Source: CAD feature listing. Evaluate the final solid. Frame: model axes, mm. A direction names the side the tool comes from. Coordinates: 2 decimals unless noted, no trailing zeros. Write each loop counter-clockwise with the first axis right and the second up, starting at its lowest first coordinate (ties: lowest second). Pieces come first, ordered by that corner, then holes. Notation, with made-up numbers: (-25.75, -25) - (-17.75, -25) arc R26 cw to (-17.75, -10) - close; hole circle Ø9 at (55.25, -19). An arc over 180 degrees is marked (long way). One line per question, with ' | ' between items. Start each with the question number.
Q1. Cut plane C-C, the plane x = -18.5. Return loops of the section in (y, z), plus the area to 3 significant figures.
Q2. Draft query along Y for faces 6 (the face through (2, 23, 6.85)), 7 (the face through (-0.86, 46.1, 5.58)), 8 (the face through (-13, 49, 4.15)). Return one class per face: +Y half, -Y half, draft (parallel to the pull), parting line (faces both ways), or undercut.
Q3. Cut plane D-D, the plane z = 1.75. Return loops of the section in (x, y), plus the area to 3 significant figures.
Q4. Line query: line 1 (Z direction, x = 1.25, y = 21); line 2 (X direction, y = 37, z = 4); line 3 (Y direction, x = -10, z = 9.5). Output: solid intervals per line, ascending.
Q5. Contact query for flat-ended pins moving along their axis: P1, Ø3.5, axis at x = -14, z = 5, coming from the -Y side; P2, Ø3.5, axis at y = 32.5, z = 8, coming from the -X side. Output: stop coordinate, or through.
Q6. Cut plane B-B, the plane z = 5.5. Give the number of separate pieces and of enclosed holes in the cut face, plus the area to 3 significant figures.
Q7. Cut plane A-A, the plane y = 35. Return loops of the section in (x, z), plus the area to 3 significant figures.
Q8. Access query for faces 1 (the face through (1.5, 44, 5.5)), 2 (the face through (0, 22, 3)), 3 (the face through (0.4, 33.6, 11)), 4 (the face through (-26.1, 48.48, 0.86)), 5 (the face through (-23.5, 48.5, 5.5)). Directions: +Z, -Z, +X, -X, +Y, -Y. A direction counts if a zero-diameter tool reaches every point of the face in a straight line with its end or side. Return the directions, or none.
```python
from build123d import *

# Parameters (mm, degrees)
BOSS_EXTRUDE1_DEPTH = 11
CUT_EXTRUDE1_DEPTH  = 60.338014797
CUT_EXTRUDE2_DEPTH  = 58.879184514
FILLET1_R           = 3
FILLET2_R           = 3


with BuildPart() as part:
    # Sketch1 → Boss-Extrude1 (new body)
    with BuildSketch(Plane.XY):
        Polygon((0, 0), (3, 0), (3, 50), (-27, 50), (-27, 47), (0, 47), align=None)
    extrude(amount=BOSS_EXTRUDE1_DEPTH)

    # Sketch6 → Cut-Extrude1 (cut, through all)
    with BuildSketch(Plane(origin=(3, 0, 0), x_dir=(0, 0, -1), z_dir=(1, 0, 0))):
        with BuildLine():
            Line((-4.15, 42.65), (-4.15, 4.85))
            ThreePointArc((-4.15, 4.85), (-5.5, 3.5), (-6.85, 4.85))
            Line((-6.85, 4.85), (-6.85, 42.65))
            ThreePointArc((-6.85, 42.65), (-5.5, 44), (-4.15, 42.65))
        make_face()
    extrude(amount=-CUT_EXTRUDE1_DEPTH, mode=Mode.SUBTRACT)

    # Sketch7 → Cut-Extrude2 (cut, through all)
    with BuildSketch(Plane(origin=(0, 50, 0), x_dir=(1, 0, 0), z_dir=(0, 1, 0))):
        with BuildLine():
            Line((-22.15, -4.15), (-4.35, -4.15))
            ThreePointArc((-4.35, -4.15), (-3, -5.5), (-4.35, -6.85))
            Line((-4.35, -6.85), (-22.15, -6.85))
            ThreePointArc((-22.15, -6.85), (-23.5, -5.5), (-22.15, -4.15))
        make_face()
    extrude(amount=-CUT_EXTRUDE2_DEPTH, mode=Mode.SUBTRACT)

    # Fillet1
    fillet1_edges = [part.edges().sort_by_distance(p)[0] for p in [
        (0, 47, 5.5),
    ]]
    fillet(fillet1_edges, radius=FILLET1_R - 0.0001)  # a hair under: the kernel refuses the full size

    # Fillet2
    fillet2_edges = [part.edges().sort_by_distance(p)[0] for p in [
        (-27, 48.5, 11),
        (-27, 48.5, 0),
        (1.5, 0, 0),
        (1.5, 0, 11),
    ]]
    fillet(fillet2_edges, radius=FILLET2_R)


solid = part.part
```
Reply:
1) outline: (47, 0) - (50, 0) - (50, 4.15) - (47, 4.15) - close; (47, 6.85) - (50, 6.85) - (50, 11) - (47, 11) - close | area: 24.9 mm^2
2) face 6: undercut | face 7: -Y half | face 8: draft
3) outline: (-26.73, 47) - (-3, 47) arc R3 cw to (0, 44) - (0, 0.27) - (3, 0.27) - (3, 50) - (-26.73, 50) - close | area: 231 mm^2
4) line 1: z = 0 to 4.15, 6.85 to 11 | line 2: x = 0 to 3 | line 3: y = 47 to 50
5) P1: stops at y = 47 | P2: stops at x = 0
6) separate pieces: 3 | enclosed holes: 0 | area: 49.9 mm^2
7) outline: (0, 0) - (3, 0) - (3, 4.15) - (0, 4.15) - close; (0, 6.85) - (3, 6.85) - (3, 11) - (0, 11) - close | area: 24.9 mm^2
8) face 1: +X, -X | face 2: +Z, -Z, -X, -Y | face 3: +Z, +X, -X, +Y, -Y | face 4: -Z, -X, +Y, -Y | face 5: +Y, -Y
